Model file for the job. Use its own axes, mm. Face numbers are marked on the shaded views. A direction names the side the tool comes from. Coordinates: 2 decimals unless noted, no trailing zeros. Order: outer loops, then holes, each group sorted by start corner. A loop starts at its lowest first (then second) coordinate and runs counter-clockwise, first axis right, second up. Notation, with made-up numbers: M 52,29.25 L 70,29.25 A32 ccw 70,60.25 Z; hole C 10,27.25 d3. An arc over 180 degrees is marked long. Return JSON: item names as keys, results as strings.
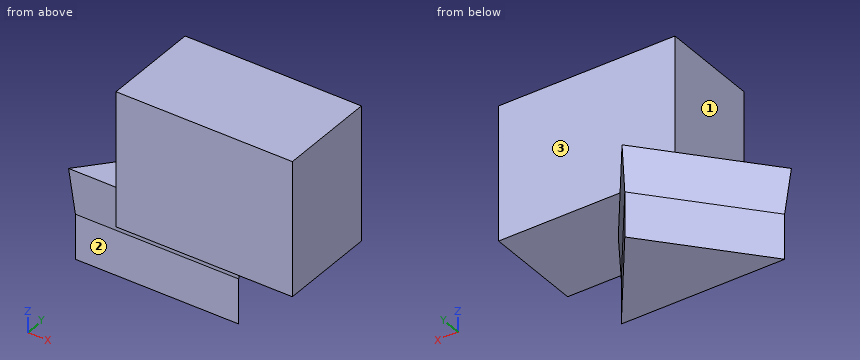
```python
from build123d import *

# Parameters (mm, degrees)
F1_DEPTH      = 25.4
F1_TAPER      = -3
F1_DEPTH_BACK = 25.4
F2_W          = 100.148499012
F2_H          = 55.9419505298
F3_DEPTH      = 76.2


with BuildPart() as f1:
    # F0 (on Top) → F1 (new body, two sides)
    with BuildSketch(Plane.XY) as f1_sk:
        Polygon((-92.7592143416, 0), (0, 0), (-42.4239225686, 57.6683394611), align=None)
    extrude(amount=F1_DEPTH, taper=F1_TAPER)
    extrude(f1_sk.sketch, amount=-F1_DEPTH_BACK)

    # F2 (on face) → F3 (join)
    with BuildSketch(Plane.XY.offset(25.4)):
        Rectangle(F2_W, F2_H)
    extrude(amount=F3_DEPTH)


solid = f1.part
```
Item 1: Saw through at C-C (x = 5.5). Write the cut outline in (y, z).
Check result:
{"outline": "M -27.97,25.4 L 27.97,25.4 L 27.97,101.6 L -27.97,101.6 Z"}
Item 2: Drop flat-ended pins along their axis: pin 1 Ø6 at (x, y) = (-76, -6) entering from +Z (3 decimals); pin 2 Ø8 at (y, z) = (19.5, 61) entering from -X; pin 3 Ø1 at (x, y) = (-53.5, 18.5) entering from +Z; pin 4 Ø2 at (x, y) = (17.5, -10) entering from -Z. Give the stop position or say it passes through.
Check result:
{"pin 1": "passes through", "pin 2": "stops at x = -50.07", "pin 3": "stops at z = 25.4", "pin 4": "stops at z = 25.4"}
Item 3: Wall check: line 1 (X direction, y = 17, z = 72); line 2 (Y direction, x = 30.5, z = 52.5); line 3 (Z direction, x = 31, y = 17). Give the ranges that are in metal, low to high.
Check result:
{"line 1": "x = -50.07 to 50.07", "line 2": "y = -27.97 to 27.97", "line 3": "z = 25.4 to 101.6"}
Item 4: 3-axis set-ups, long thin cutter, end or side, ignore diameter. For the marked faces 1, 2 and 3: which of +Z, -Z, +X, -X, +Y, -Y reach the whole face in a straight line?
Check result:
{"face 1": "+Z, -X, +Y, -Y", "face 2": "-Z, +X, -X, -Y", "face 3": "+Z, +X, -X, +Y"}
Item 5: Saw through at A-A (z = -2.5). Write the cut outline in (x, y).
Check result:
{"outline": "M -92.76,0 L 0,0 L -42.42,57.67 Z"}
Item 6: Saw through at B-B (y = -3.5). Write the cut outline in (x, z), and give its area (3 significant figures).
Check result:
{"outline": "M -50.07,25.4 L 50.07,25.4 L 50.07,101.6 L -50.07,101.6 Z", "area": "7,630 mm2"}
